```python
from build123d import *

# Parameters (mm, degrees)
BOSS_EXTRUDE1_DEPTH            = 30
HOLE_FOR_M5_300_SC_NUTS_SP_1_D = 10
HOLE_FOR_M5_300_SC_NUTS_SP_2_D = 3.5


with BuildPart() as part:
    # Sketch1 → Boss-Extrude1 (new body)
    with BuildSketch(Plane.XY):
        Polygon((-7.897485035, 31.347562808), (-7.897485035, 2.347562808), (14.102514965, 2.347562808), (14.102514965, -0.652437192), (-10.897485035, -0.652437192), (-10.897485035, 31.347562808), align=None)
    extrude(amount=BOSS_EXTRUDE1_DEPTH)

    # Hole for M5 300® SC Nuts (SP)1 (through all)
    with Locations(Plane(origin=(-7.897485035, 0, 0), x_dir=(0, 0, -1), z_dir=(1, 0, 0))):
        with Locations((-15, 18.347562808)):
            Hole(HOLE_FOR_M5_300_SC_NUTS_SP_1_D / 2)

    # Hole for M5 300® SC Nuts (SP)2 (through all)
    with Locations(Plane(origin=(-7.897485035, 0, 0), x_dir=(0, 0, -1), z_dir=(1, 0, 0))):
        with Locations((-7, 18.347562808), (-23, 18.347562808), (-15, 10.347562808)):
            Hole(HOLE_FOR_M5_300_SC_NUTS_SP_2_D / 2)


solid = part.part
```
Verification items for the finished model (mm, model axes). A direction names the side the tool comes from. Coordinates: 2 decimals unless noted, no trailing zeros. Write each loop counter-clockwise with the first axis right and the second up, starting at its lowest first coordinate (ties: lowest second). Pieces come first, ordered by that corner, then holes. Notation, with made-up numbers: M -28.75,40 L 24.25,40 A31 ccw 24.25,66 Z; hole C 29.25,18 d7. An arc over 180 degrees is marked long. Answer as a JSON object with one key per item and string values. Group by question number.
(1) Tool access check on faces 1 (the face through (-7.897, 14, 18)), 2 (the face through (-10.897, 12, 11)). Record the directions out of +Z, -Z, +X, -X, +Y, -Y that give a thin tool (end or side, any length) a straight path to the whole face; none if there is none.
(2) Cross-section at A-A, the plane z = 15. Record the cut outline in (x, y), and give its area (4 significant figures).
(3) Gauge pin test, flat ends, axial feed: pin 1 (10 mm diameter, centred on y = 21, z = 23.5, fed in from +X); pin 2 (3 mm diameter, centred on y = 18.35, z = 7, fed in from +X); pin 3 (6.5 mm diameter, centred on x = 0, z = 18, fed in from +Y). Record the tip position at first contact, or that the pin passes through.
(4) Material ranges on line 1 (Y direction, x = -10.2, z = 15); line 2 (Y direction, x = -9.7, z = 23); line 3 (X direction, y = 22.5, z = 23.75), recorded low to high.
(5) Cross-section at C-C, the plane y = 15. Record the cut outline in (x, z), and give its area (3 significant figures).
(6) Cross-section at D-D, the plane x = 8.5. Record the cut outline in (y, z).
(7) Release check for a two-part mould opening along Y. For faces 3 (the face through (-9.418, 20.083, 6.772)), 4 (the face through (14.103, 1, 15)), 5 (the face through (3, 2.348, 15)) record: +Y half, -Y half, draft (parallel to the pull), parting line (faces both ways), or undercut.
(8) Cross-section at B-B, the plane z = 7. Record the cut outline in (x, y).
Reply:
{
 "1": {"face 1": "+Z, -Z, +X, +Y", "face 2": "+Z, -Z, -X, +Y, -Y"},
 "2": {"outline": "M -10.9,-0.65 L 14.1,-0.65 L 14.1,2.35 L -7.9,2.35 L -7.9,8.6 L -10.9,8.6 Z; M -10.9,12.1 L -7.9,12.1 L -7.9,13.35 L -10.9,13.35 Z; M -10.9,23.35 L -7.9,23.35 L -7.9,31.35 L -10.9,31.35 Z", "area": "121.5 mm²"},
 "3": {"pin 1": "x = -7.9", "pin 2": "through", "pin 3": "y = 2.35"},
 "4": {"line 1": "-0.65 to 8.6, 12.1 to 13.35, 23.35 to 31.35", "line 2": "-0.65 to 16.6, 20.1 to 31.35", "line 3": "-10.9 to -7.9"},
 "5": {"outline": "M -10.9,0 L -7.9,0 L -7.9,11.29 L -10.9,11.29 Z; M -10.9,18.71 L -7.9,18.71 L -7.9,30 L -10.9,30 Z", "area": "67.7 mm²"},
 "6": {"outline": "M -0.65,0 L 2.35,0 L 2.35,30 L -0.65,30 Z"},
 "7": {"face 3": "undercut", "face 4": "draft", "face 5": "+Y half"},
 "8": {"outline": "M -10.9,-0.65 L 14.1,-0.65 L 14.1,2.35 L -7.9,2.35 L -7.9,16.6 L -10.9,16.6 Z; M -10.9,20.1 L -7.9,20.1 L -7.9,31.35 L -10.9,31.35 Z"}
}
